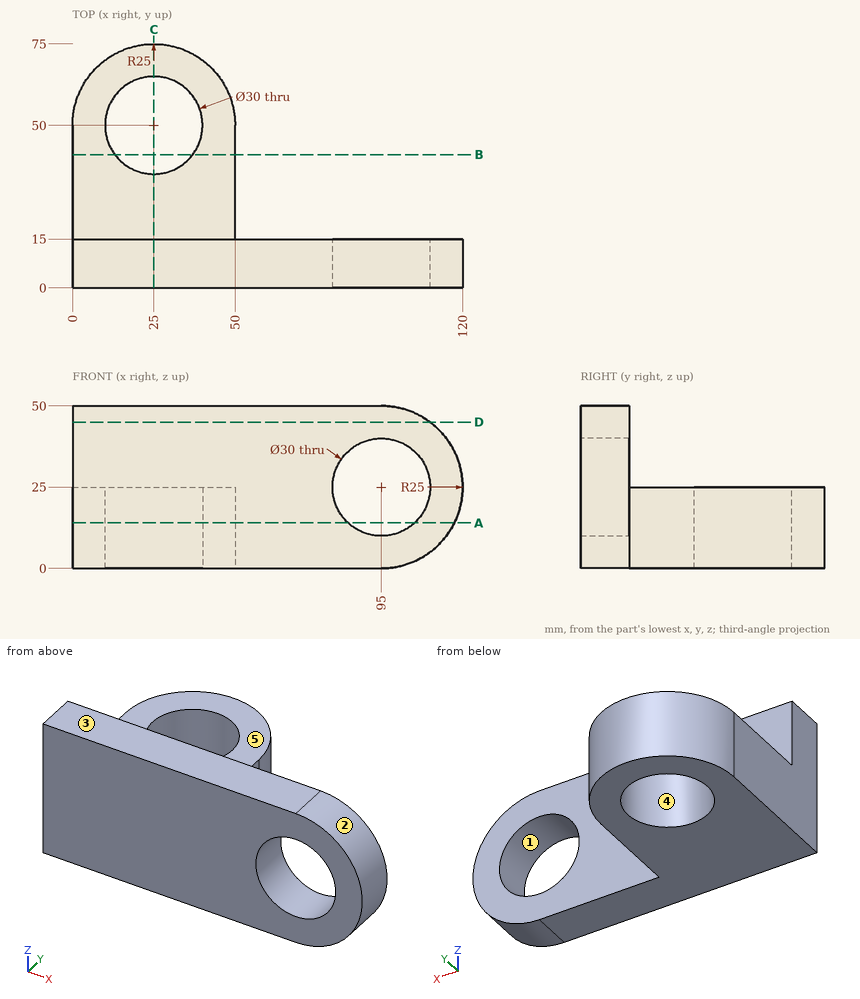
Print and shaded views of the part. All mm, measured from the part's lowest x, y and z. A direction names the side the tool comes from. Give positions to 0.01 mm unless a question says otherwise; leave off trailing zeros. Loops run counter-clockwise (first coordinate to the right, second up) from the corner with the lowest first, then second, coordinate; pieces in that order, holes last. Notation, with made-up numbers: (31, 41.25) - (35, 41.25) arc R33 ccw to (35, 79.25) - close; hole circle Ø3 at (-23, 87.25). An arc over 180 degrees is marked (long way). Use a Markdown table: item, result.
(1) Wall check: line 1 along X through (y, z) = (10.75, 25); line 2 along Y through (x, z) = (25, 9); line 3 along X through (y, z) = (49.5, 23). Give the ranges that are in metal, low to high.
Taken from the geometry:
| item | result |
|---|---|
| line 1 | 0 to 80, 110 to 120 |
| line 2 | 0 to 35, 65 to 75 |
| line 3 | 0 to 10.01, 39.99 to 50 |
(2) Drop flat-ended pins along their axis: pin 1 Ø12 at (y, z) = (28, 22) entering from -X; pin 2 Ø4 at (x, y) = (13, 57) entering from +Z; pin 3 Ø7.5 at (y, z) = (39.5, 8) entering from +X; pin 4 Ø1 at (x, z) = (23, 41.5) entering from +Y. Give the stop position or say it passes through.
Taken from the geometry:
| item | result |
|---|---|
| pin 1 | x = 0 |
| pin 2 | z = 25 |
| pin 3 | x = 50 |
| pin 4 | y = 15 |
(3) Band-saw the part on A-A (z = 14). Give the cut face in (x, y), and give its area (3 significant figures).
Taken from the geometry:
| item | result |
|---|---|
| outline | (0, 0) - (84.8, 0) - (84.8, 15) - (50, 15) - (50, 50) arc R25 ccw to (0, 50) - close; (105.2, 0) - (117.45, 0) - (117.45, 15) - (105.2, 15) - close; hole circle Ø30 at (25, 50) |
| area | 3,480 mm2 |
(4) Band-saw the part on C-C (x = 25). Give the cut face in (y, z).
Taken from the geometry:
| item | result |
|---|---|
| outline | (0, 0) - (35, 0) - (35, 25) - (15, 25) - (15, 50) - (0, 50) - close; (65, 0) - (75, 0) - (75, 25) - (65, 25) - close |
(5) Band-saw the part on D-D (z = 45). Give the cut face in (x, y).
Taken from the geometry:
| item | result |
|---|---|
| outline | (0, 0) - (110, 0) - (110, 15) - (0, 15) - close |
(6) Which spindle directions (+Z, -Z, +X, -X, +Y, -Y) get a long thin tool onto all of the face, cutting with end or side? Do the marked faces 4 and 5. Say none if no direction does.
Taken from the geometry:
| item | result |
|---|---|
| face 4 | +Z, -Z |
| face 5 | +Z, +X, -X, +Y |
(7) Pull direction X, two halves, no side cores. Call the marked faces 1, 2 and 3: +X half, -X half, draft (parallel to the pull), parting line (faces both ways), or undercut.
Taken from the geometry:
| item | result |
|---|---|
| face 1 | undercut |
| face 2 | +X half |
| face 3 | draft |
(8) Band-saw the part on B-B (y = 41). Give the cut face in (x, z), and give its area (3 significant figures).
Taken from the geometry:
| item | result |
|---|---|
| outline | (0, 0) - (13, 0) - (13, 25) - (0, 25) - close; (37, 0) - (50, 0) - (50, 25) - (37, 25) - close |
| area | 650 mm2 |
